Input: dimensioned drawing with shaded views. Units: mm. Origin: part minimum x, y, z. A direction names the side the tool comes from. Round coordinates to 2 decimals unless told otherwise and drop trailing zeros. Loops run counter-clockwise (first coordinate to the right, second up) from the corner with the lowest first, then second, coordinate; pieces in that order, holes last.
1) Ray query, line 1 along Y through (x, z) = (50, 69) (1 decimal); line 2 along X through (y, z) = (5.5, 59.5) (1 decimal); line 3 along X through (y, z) = (3, 13.5) (1 decimal). Return the intervals inside material, ascending.
2) Section D-D, the plane z = 61.5. Return loops of the section in (x, y) (1 decimal).
3) Section C-C, the plane y = 3.25. Return loops of the section in (x, z), and give its area (3 significant figures).
4) Access query for the marked faces 1 and 2. Directions: +Z, -Z, +X, -X, +Y, -Y. A direction counts if a zero-diameter tool reaches every point of the face in a straight line with its end or side. Return the directions, or none.
5) First-contact query: pin 1 (2 mm diameter, centred on x = 23, y = 1.5, fed in from -Z); pin 2 (3 mm diameter, centred on x = 29.5, y = 1.5, fed in from -Z); pin 3 (2 mm diameter, centred on y = 3.5, z = 64, fed in from -X). Flat tips, straight axial feed; report the tip coordinate or a pass-through.
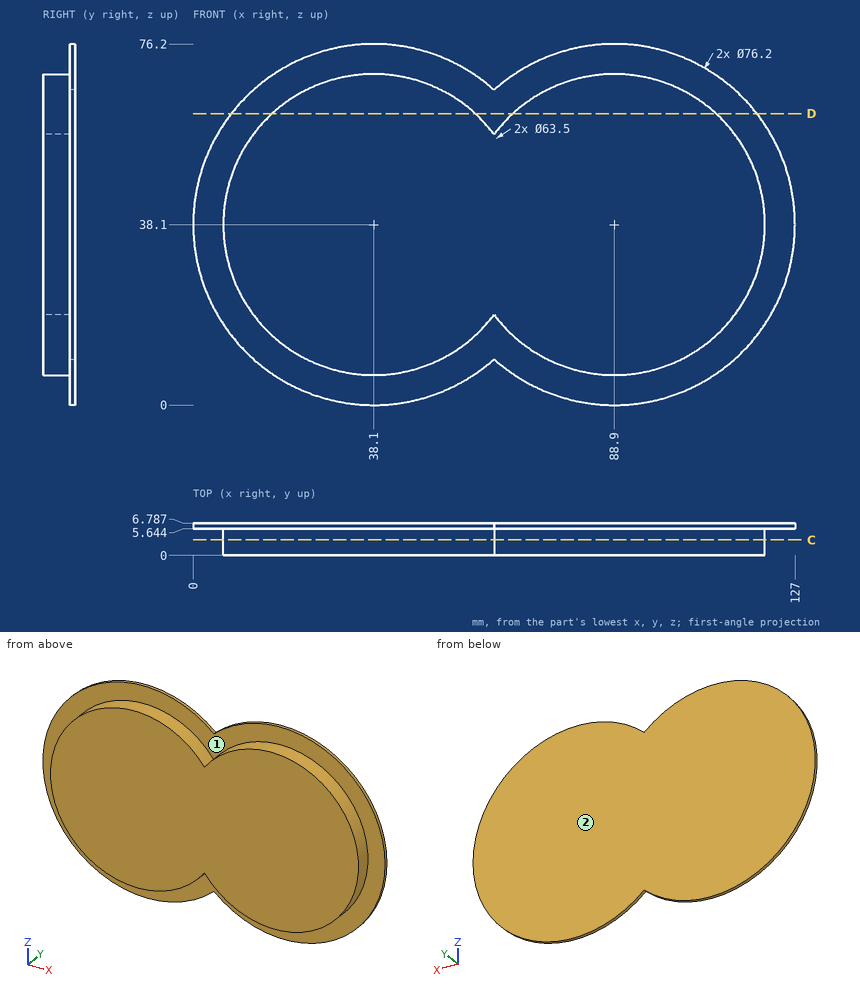
Final values:
1. line 1: y = 5.6 to 6.8
1. line 2: x = 14.6 to 61.6, 65.4 to 112.4
1. line 3: x = 18 to 58.2, 68.8 to 109
2. outline: (8, 5.6) - (16.6, 5.6) - (16.6, 0) - (59.6, 0) - (59.6, 5.6) - (67.4, 5.6) - (67.4, 0) - (110.4, 0) - (110.4, 5.6) - (119, 5.6) - (119, 6.8) - (8, 6.8) - close
3. outline: (63.5, 19.05) arc R31.75 ccw (long way) to (63.5, 57.15) arc R31.75 ccw (long way) to start
3. area: 6,000 mm2
4. face 1: -Y
4. face 2: +Z, -Z, +X, -X, +Y
5. pin 1: stops at z = 9.65
5. pin 2: stops at z = 7.15
5. pin 3: stops at x = 18.4
